from build123d import *

# Parameters (mm, degrees)
SKETCH1_R           = 2.5
BOSS_EXTRUDE1_DEPTH = 4.5
SKETCH2_R           = 0.5
BOSS_EXTRUDE2_DEPTH = 25


with BuildPart() as part:
    # Sketch1 → Boss-Extrude1 (new body, symmetric)
    with BuildSketch(Plane(origin=(0, 0, 0), x_dir=(1, 0, 0), z_dir=(0, 1, 0))):
        Circle(SKETCH1_R)
    extrude(amount=BOSS_EXTRUDE1_DEPTH, both=True)

    # Sketch2 → Boss-Extrude2 (add)
    with BuildSketch(Plane(origin=(0, 4.5, 0), x_dir=(1, 0, 0), z_dir=(0, 1, 0))):
        Circle(SKETCH2_R)
    boss_extrude2 = extrude(amount=BOSS_EXTRUDE2_DEPTH)

    # Mirror4: Boss-Extrude2 across plane
    add(boss_extrude2.mirror(Plane.ZX))


solid = part.part
Here's how the part is built. I have some questions about the finished solid (model axes, mm). A direction names the side the tool comes from. Coordinates: 2 decimals unless noted, no trailing zeros. Loops run counter-clockwise (first coordinate to the right, second up) from the corner with the lowest first, then second, coordinate; pieces in that order, holes last.
1. For P1, Ø1.5, axis at y = 21.5, z = 1, coming from the +X side; P2, Ø1.5, axis at x = -0.5, y = -10.5, coming from the -Z side; P3, Ø2, axis at x = -1.5, z = 1, coming from the +Y side, each with a flat end and sliding along its axis, tell me the tip position at first contact or that it passes through.
2. I need wall thicknesses on L1, parallel to Y at x = 1.85, z = 1.45; L2, parallel to X at y = 20.5, z = 0.4; L3, parallel to X at y = 3.5, z = 1.2. Which ranges of each line are inside material? Lowest first, please.
3. Imagine slicing it at B-B, the plane x = 0. Please give me the cut outline in (y, z), and give its area (3 significant figures).
4. For faces 1 (the cylindrical face through (-0.108, -16.825, 0.488)), 2 (the cylindrical face through (-0.108, 16.825, 0.488)), 3 (the flat face through (0, 29.5, 0)), which set-ups out of +Z, -Z, +X, -X, +Y, -Y let a thin tool reach every point of the face, with its end or its side?
5. Imagine slicing it at A-A, the plane z = 0. Please give me the cut outline in (x, y).
6. Imagine slicing it at C-C, the plane y = -5. Please give me the cut outline in (x, z).
Taken from the geometry:
1. P1: stops at x = 0.43
1. P2: stops at z = -0.5
1. P3: stops at y = 4.5
2. L1: y = -4.5 to 4.5
2. L2: x = -0.3 to 0.3
2. L3: x = -2.19 to 2.19
3. outline: (-29.5, -0.5) - (-4.5, -0.5) - (-4.5, -2.5) - (4.5, -2.5) - (4.5, -0.5) - (29.5, -0.5) - (29.5, 0.5) - (4.5, 0.5) - (4.5, 2.5) - (-4.5, 2.5) - (-4.5, 0.5) - (-29.5, 0.5) - close
3. area: 95.0 mm2
4. face 1: -Y
4. face 2: +Y
4. face 3: +Z, -Z, +X, -X, +Y
5. outline: (-2.5, -4.5) - (-0.5, -4.5) - (-0.5, -29.5) - (0.5, -29.5) - (0.5, -4.5) - (2.5, -4.5) - (2.5, 4.5) - (0.5, 4.5) - (0.5, 29.5) - (-0.5, 29.5) - (-0.5, 4.5) - (-2.5, 4.5) - close
6. outline: circle Ø1 at (0, 0)
